```python
from build123d import *

# Parameters (mm, degrees)
SKETCH1_R           = 1.25
BOSS_EXTRUDE1_DEPTH = 3.5
BOSS_EXTRUDE2_DEPTH = 8
SKETCH3_R           = 1.25
CUT_EXTRUDE1_DEPTH  = 4.8
SKETCH5_OUTSIDE_W   = 34.18
SKETCH5_OUTSIDE_H   = 34.876
SKETCH5_OUTSIDE_R   = 2.25
CUT_EXTRUDE2_DEPTH  = 12.5
CUT_EXTRUDE2_TAPER  = 45
SKETCH6_OUTSIDE_W   = 27.18
SKETCH6_OUTSIDE_H   = 27.876
SKETCH6_OUTSIDE_R   = 2.25
CUT_EXTRUDE3_DEPTH  = 9
CUT_EXTRUDE3_TAPER  = 45
CHAMFER1_SIZE       = 0.3
CHAMFER1_SIZE2      = 0.357526078


with BuildPart() as part:
    # Sketch1 → Boss-Extrude1 (new body)
    with BuildSketch(Plane(origin=(0, 0, 0), x_dir=(1, 0, 0), z_dir=(0, 1, 0))):
        Circle(SKETCH1_R)
    extrude(amount=BOSS_EXTRUDE1_DEPTH)

    # Sketch2 → Boss-Extrude2 (add)
    with BuildSketch(Plane(origin=(0, 3.5, 0), x_dir=(1, 0, 0), z_dir=(0, 1, 0))):
        Polygon((2.25, -1.299038106), (2.25, 1.299038106), (0, 2.598076211), (-2.25, 1.299038106), (-2.25, -1.299038106), (0, -2.598076211), align=None)
    extrude(amount=BOSS_EXTRUDE2_DEPTH)

    # Sketch3 → Cut-Extrude1 (cut)
    with BuildSketch(Plane(origin=(0, 11.5, 0), x_dir=(1, 0, 0), z_dir=(0, 1, 0))):
        Circle(SKETCH3_R)
    extrude(amount=-CUT_EXTRUDE1_DEPTH, mode=Mode.SUBTRACT)

    # Sketch5 outside → Cut-Extrude2 (cut, through all)
    with BuildSketch(Plane(origin=(0, 11.5, 0), x_dir=(1, 0, 0), z_dir=(0, 1, 0))):
        Rectangle(SKETCH5_OUTSIDE_W, SKETCH5_OUTSIDE_H)
        Circle(SKETCH5_OUTSIDE_R, mode=Mode.SUBTRACT)
    extrude(amount=-CUT_EXTRUDE2_DEPTH, taper=CUT_EXTRUDE2_TAPER, mode=Mode.SUBTRACT)

    # Sketch6 outside → Cut-Extrude3 (cut, through all)
    with BuildSketch(Plane.XZ.offset(-3.5)):
        Rectangle(SKETCH6_OUTSIDE_W, SKETCH6_OUTSIDE_H)
        Circle(SKETCH6_OUTSIDE_R, mode=Mode.SUBTRACT)
    extrude(amount=-CUT_EXTRUDE3_DEPTH, taper=CUT_EXTRUDE3_TAPER, mode=Mode.SUBTRACT)

    # Chamfer1
    chamfer1_edges = [part.edges().sort_by_distance(p)[0] for p in [
        (-1.25, 0, 0),
    ]]
    chamfer1_side = [part.faces().sort_by_distance(p)[0] for p in [
        (0, 0, 0),
    ]]
    chamfer(chamfer1_edges, length=CHAMFER1_SIZE, length2=CHAMFER1_SIZE2, reference=chamfer1_side[0])


solid = part.part
```
Read the model definition and answer for the solid it produces. Units are mm, in the model's axes. A direction names the side the tool comes from. Coordinates: 2 decimals unless noted, no trailing zeros. Loops run counter-clockwise (first coordinate to the right, second up) from the corner with the lowest first, then second, coordinate; pieces in that order, holes last. Notation, with made-up numbers: (82, -13) -> (122, -13) arc R14 cw to (122, 14) -> close; hole circle Ø1 at (66.5, -32.5). An arc over 180 degrees is marked (long way). Return JSON: item names as keys, results as strings.
Item 1: Find section A-A (y = 10.5). Determine the outline of the cut face in (x, z), plus the area to 3 significant figures.
Answers:
{"outline": "(-2.25, -1.3) -> (0, -2.6) -> (2.25, -1.3) -> (2.25, 1.3) -> (0, 2.6) -> (-2.25, 1.3) -> close; hole circle Ø2.5 at (0, 0)", "area": "12.6 mm2"}
Item 2: For faces 5 (the flat face through (1, 3.5, 1)), 6 (the conical face through (2.05, 3.62, 1.19)), determine the directions among +Z, -Z, +X, -X, +Y, -Y from which every point of the face is accessible in a straight line to the end or side of a thin tool.
Answers:
{"face 5": "-Y", "face 6": "+Z, +X, -Y"}
Item 3: Find the intervals of material crossed by probe 1 along X at (y, z) = (7.95, 0); probe 2 along X at (y, z) = (8.25, 0.55); probe 3 along Y at (x, z) = (0.6, -0.45), in increasing order.
Answers:
{"probe 1": "x = -2.25 to -1.25, 1.25 to 2.25", "probe 2": "x = -2.25 to -1.12, 1.12 to 2.25", "probe 3": "y = 0 to 6.7"}
Item 4: Flat-ended cylindrical pins translate along their axes: P1, Ø2, axis at x = 0, z = 0, coming from the +Y side; P2, Ø1, axis at x = -1, y = 5, coming from the +Z side; P3, Ø2, axis at x = -0.5, z = 0, coming from the -Y side; P4, Ø1, axis at x = -1.5, y = 5, coming from the -Z side. Find the tip coordinate at first contact, or state that the pin passes through.
Answers:
{"P1": "stops at y = 6.7", "P2": "stops at z = 2.31", "P3": "stops at y = 0", "P4": "stops at z = -2.02"}
Item 5: For a pull along Z with two mould halves and no side action, classify faces 1 (the flat face through (0, 0, 0)), 2 (the flat face through (0, 6.7, 0)), 3 (the conical face through (-2.05, 3.62, -1.19)), 4 (the flat face through (1.109, 7.444, 1.958)) as +Z half, -Z half, draft (parallel to the pull), parting line (faces both ways), or undercut.
Answers:
{"face 1": "draft", "face 2": "undercut", "face 3": "-Z half", "face 4": "+Z half"}
Item 6: Find section B-B (y = 6.5). Determine the outline of the cut face in (x, z), plus the area to 3 significant figures.
Answers:
{"outline": "(-2.25, -1.3) -> (0, -2.6) -> (2.25, -1.3) -> (2.25, 1.3) -> (0, 2.6) -> (-2.25, 1.3) -> close", "area": "17.5 mm2"}
Item 7: Find section C-C (y = 2.25). Determine the outline of the cut face in (x, z).
Answers:
{"outline": "circle Ø2.5 at (0, 0)"}
